Geometry check sheet. Reference: drawing and pictorial views, mm from the part's lowest x, y, z. Round coordinates to 2 decimals unless told otherwise and drop trailing zeros. Order: outer loops, then holes, each group sorted by start corner. A loop starts at its lowest first (then second) coordinate and runs counter-clockwise, first axis right, second up.
Q1. Cross-section at C-C on y = 0.75. Give the number of separate pieces and of enclosed holes in the cut face.
Q2. Depth check by flat-ended pin: P1, Ø0.5, axis at y = 0.5, z = 33, coming from the +X side; P2, Ø2.5, axis at x = 6.35, z = 82.55, coming from the -Y side; P3, Ø5, axis at x = 178, z = 70, coming from the +Y side. Enter the tip coordinate at first touch or a pass-through.
Q3. Scan lines: probe 1 along Z at (x, y) = (6.35, 1.2) (1 decimal); probe 2 along X at (y, z) = (1.3, 6.5); probe 3 along Z at (x, y) = (35, 0.9). Record each from-to range of solid material in increasing order.
Q4. Cross-section at D-D on z = 62. Record the cut outline in (x, y).
Q5. Cross-section at B-B on z = 82.55. Record the cut outline in (x, y) (1 decimal).
Q6. Cross-section at A-A on x = 87. Record the cut outline in (y, z).
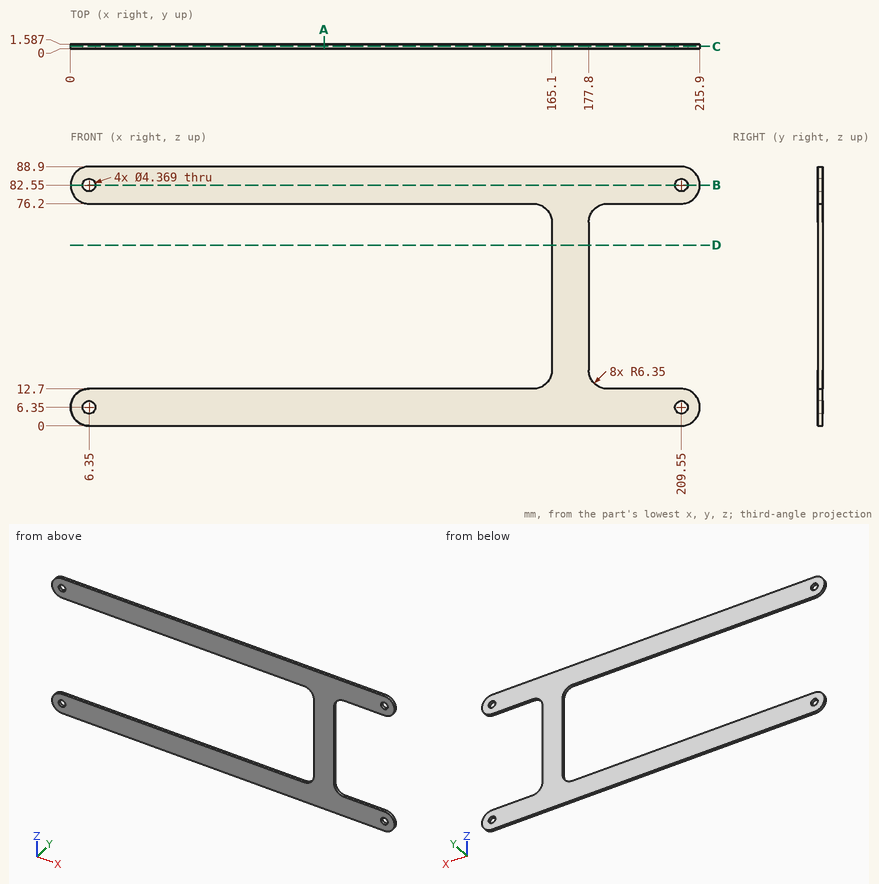
Results found:
1. separate pieces: 1
1. enclosed holes: 4
2. P1: stops at x = 177.8
2. P2: passes through
2. P3: stops at y = 1.59
3. probe 1: z = 0 to 4.2, 8.5 to 12.7, 76.2 to 80.4, 84.7 to 88.9
3. probe 2: x = 0 to 4.17, 8.53 to 207.37, 211.73 to 215.9
3. probe 3: z = 0 to 12.7, 76.2 to 88.9
4. outline: (165.1, 0) - (177.8, 0) - (177.8, 1.59) - (165.1, 1.59) - close
5. outline: (0, 0) - (4.2, 0) - (4.2, 1.6) - (0, 1.6) - close; (8.5, 0) - (207.4, 0) - (207.4, 1.6) - (8.5, 1.6) - close; (211.7, 0) - (215.9, 0) - (215.9, 1.6) - (211.7, 1.6) - close
6. outline: (0, 0) - (1.59, 0) - (1.59, 12.7) - (0, 12.7) - close; (0, 76.2) - (1.59, 76.2) - (1.59, 88.9) - (0, 88.9) - close
